Design review of the part built by this model. Coordinates are the model's own, in mm. A direction names the side the tool comes from. Coordinates: 2 decimals unless noted, no trailing zeros. Loops run counter-clockwise (first coordinate to the right, second up) from the corner with the lowest first, then second, coordinate; pieces in that order, holes last.
Q1. Machinability: for faces 5 (the face through (13.29, 2.96, 9.91)), 6 (the face through (0, 6, 37)), 7 (the face through (20, 7, 22.74)), 8 (the face through (19.74, 7.4, 20.68)), 9 (the face through (-16, 3, 6.5)), which of the approach directions +Z, -Z, +X, -X, +Y, -Y give a long, thin tool a straight path to every point of the face, cutting with its end or side? Answer none if there is none.
Q2. Wall thickness on probe 1 along X at (y, z) = (3.2, 22.5); probe 2 along X at (y, z) = (1.75, 36); probe 3 along X at (y, z) = (4.5, 19.5): over which ranges is each line inside the solid? List them lowest first.
Q3. Add section D-D on y = 13. Give the boundary of the cut face in (x, z).
Q4. Add section A-A on z = 28.5. Give the boundary of the cut face in (x, y), and give its area (3 significant figures).
Q5. Add section B-B on x = 20.5. Give the boundary of the cut face in (y, z), and give its area (3 significant figures).
Q6. Draft analysis for pull direction Z (two halves, no side actions). For faces 1 (the face through (22, 15, 14)), 2 (the face through (19.28, 7.4, 13.86)), 3 (the face through (0, 3, 33)), 4 (the face through (-7.96, 2.96, 35.15)), state which applies: released by +Z, released by -Z, zero draft, split by the parting line, or undercut.
Q7. Add section C-C on z = 19.69. Give the boundary of the cut face in (x, y), and give its area (4 significant figures).
Q8. For P1, Ø1.9, axis at x = -16.5, y = 3, coming from the -Z side; P2, Ø12, axis at x = -8, z = 27, coming from the +Y side; P3, Ø1.5, axis at y = 8.5, z = 29.5, coming from the -X side; P4, Ø4, axis at x = 20.5, z = 19.69, coming from the +Y side, all flat-tipped, find the tip position at first contact; note any pin that passes through.
```python
from build123d import *

# Parameters (mm, degrees)
SKETCH1_R           = 0.85
BOSS_EXTRUDE1_DEPTH = 6
BOSS_EXTRUDE2_DEPTH = 15
SKETCH4_R           = 1.25
CUT_EXTRUDE2_DEPTH  = 49.187135213
CUT_EXTRUDE3_DEPTH  = 10
SKETCH7_W           = 1.75
SKETCH7_H           = 1.777688456
BOSS_EXTRUDE4_DEPTH = 6


with BuildPart() as part:
    # Sketch1 → Boss-Extrude1 (new body)
    with BuildSketch(Plane(origin=(0, 0, 0), x_dir=(1, 0, 0), z_dir=(0, 1, 0))):
        with BuildLine():
            Line((-17, -6.5), (-17, -33.5))
            Line((-17, -33.5), (-17, -39))
            Line((-17, -39), (17, -39))
            Line((17, -39), (17, -33.5))
            Line((17, -33.5), (17, -6.5))
            Line((17, -6.5), (15.25, -6.5))
            ThreePointArc((15.25, -6.5), (13.258096668, -9.951651759), (10.5, -12.828191611))
            Line((10.5, -12.828191611), (10.5, -30.5))
            Line((10.5, -30.5), (8, -30.5))
            Line((8, -30.5), (8, -33))
            Line((8, -33), (-8, -33))
            Line((-8, -33), (-8, -30.5))
            Line((-8, -30.5), (-10.5, -30.5))
            Line((-10.5, -30.5), (-10.5, -12.828191611))
            ThreePointArc((-10.5, -12.828191611), (-13.258096668, -9.951651759), (-15.25, -6.5))
            Line((-15.25, -6.5), (-17, -6.5))
        make_face()
        with Locations(Location((-13.5, -30.5, 0), (0, 0, 270))):
            Circle(SKETCH1_R, mode=Mode.SUBTRACT)
        with Locations(Location((-13.5, -22.5, 0), (0, 0, 270))):
            Circle(SKETCH1_R, mode=Mode.SUBTRACT)
        with Locations(Location((-13.5, -14.5, 0), (0, 0, 270))):
            Circle(SKETCH1_R, mode=Mode.SUBTRACT)
        with Locations(Location((-8, -36, 0), (0, 0, 270))):
            Circle(SKETCH1_R, mode=Mode.SUBTRACT)
        with Locations(Location((8, -36, 0), (0, 0, 270))):
            Circle(SKETCH1_R, mode=Mode.SUBTRACT)
        with Locations(Location((13.5, -30.5, 0), (0, 0, 270))):
            Circle(SKETCH1_R, mode=Mode.SUBTRACT)
        with Locations(Location((13.5, -22.5, 0), (0, 0, 270))):
            Circle(SKETCH1_R, mode=Mode.SUBTRACT)
        with Locations(Location((13.5, -14.5, 0), (0, 0, 270))):
            Circle(SKETCH1_R, mode=Mode.SUBTRACT)
    extrude(amount=BOSS_EXTRUDE1_DEPTH)

    # Sketch3 → Boss-Extrude2 (add)
    with BuildSketch(Plane.XZ):
        Polygon((17, 22.74), (24, 22.74), (24, 4.72), (17, 4.72), (17, 7.901808389), align=None)
    extrude(amount=-BOSS_EXTRUDE2_DEPTH)

    # Sketch4 → Cut-Extrude2 (cut, through all)
    with BuildSketch(Plane.XZ):
        with Locations(Location((20.5, 7.63, 0), (0, 0, 270))):
            Circle(SKETCH4_R)
        with Locations(Location((20.5, 13.59, 0), (0, 0, 270))):
            Circle(SKETCH4_R)
        with Locations(Location((20.5, 19.69, 0), (0, 0, 270))):
            Circle(SKETCH4_R)
    extrude(amount=-CUT_EXTRUDE2_DEPTH, mode=Mode.SUBTRACT)

    # Sketch5 → Cut-Extrude3 (cut)
    with BuildSketch(Plane.XZ):
        with BuildLine():
            Line((8, 33), (-8, 33))
            ThreePointArc((-8, 33), (-9.767766953, 32.267766953), (-10.5, 30.5))
            Line((-10.5, 30.5), (10.5, 30.5))
            ThreePointArc((10.5, 30.5), (9.767766953, 32.267766953), (8, 33))
        make_face()
    extrude(amount=-CUT_EXTRUDE3_DEPTH, mode=Mode.SUBTRACT)

    # Sketch7 → Boss-Extrude4 (add)
    with BuildSketch(Plane(origin=(0, 6, 0), x_dir=(1, 0, 0), z_dir=(0, 1, 0))):
        with Locations((16.125, -5.611155772)):
            Rectangle(SKETCH7_W, SKETCH7_H)
    extrude(amount=-BOSS_EXTRUDE4_DEPTH)


solid = part.part
```
Entries:
1. face 5: -Z, +Y, -Y
1. face 6: +Z, -Z, -X, +Y
1. face 7: +Z, +X, +Y, -Y
1. face 8: +Y, -Y
1. face 9: -Z, -X, +Y, -Y
2. probe 1: x = -17 to -14.35, -12.65 to -10.5, 10.5 to 12.65, 14.35 to 24
2. probe 2: x = -17 to -8.85, -7.15 to 7.15, 8.85 to 17
2. probe 3: x = -17 to -10.5, 10.5 to 19.26, 21.74 to 24
3. outline: (17, 4.72) - (24, 4.72) - (24, 22.74) - (17, 22.74) - close; hole circle Ø2.5 at (20.5, 7.63); hole circle Ø2.5 at (20.5, 13.59); hole circle Ø2.5 at (20.5, 19.69)
4. outline: (-17, 0) - (-10.5, 0) - (-10.5, 6) - (-17, 6) - close; (10.5, 0) - (17, 0) - (17, 6) - (10.5, 6) - close
4. area: 78.0 mm2
5. outline: (0, 4.72) - (15, 4.72) - (15, 6.38) - (0, 6.38) - close; (0, 8.88) - (15, 8.88) - (15, 12.34) - (0, 12.34) - close; (0, 14.84) - (15, 14.84) - (15, 18.44) - (0, 18.44) - close; (0, 20.94) - (15, 20.94) - (15, 22.74) - (0, 22.74) - close
5. area: 158 mm2
6. face 1: zero draft
6. face 2: undercut
6. face 3: released by -Z
6. face 4: undercut
7. outline: (-17, 0) - (-10.5, 0) - (-10.5, 6) - (-17, 6) - close; (10.5, 0) - (19.25, 0) - (19.25, 15) - (17, 15) - (17, 6) - (10.5, 6) - close; (21.75, 0) - (24, 0) - (24, 15) - (21.75, 15) - close
7. area: 145.5 mm2
8. P1: stops at z = 6.5
8. P2: stops at y = 6
8. P3: passes through
8. P4: stops at y = 15
